Can you work these out from the model? Positions are in its coordinate system, mm. A direction names the side the tool comes from. Round coordinates to 2 decimals unless told otherwise and drop trailing zeros. Order: outer loops, then holes, each group sorted by start corner. A loop starts at its lowest first (then second) coordinate and runs counter-clockwise, first axis right, second up.
Q1. If I drill on line 1 (Y direction, x = 0, z = 0.6) (3 decimals); line 2 (X direction, y = 21.5, z = 5.5); line 3 (X direction, y = 8, z = 4.25), over which ranges is the centre line in solid material (lowest first)?
Q2. If we section it at D-D (y = 8): Please give me the cut outline in (x, z).
Q3. Will this pin go through, and if not, where does the flat tip stop? P1, Ø3.5, axis at x = -3.5, y = -24.5, coming from the +Z side.
Q4. For faces 1 (the face through (2, 23, 1)), 2 (the face through (0, -30.3, 6)), 3 (the face through (1, -32.5, 4)), which set-ups out of +Z, -Z, +X, -X, +Y, -Y let a thin tool reach every point of the face, with its end or its side?
Q5. If we section it at A-A (y = -24.5): Please give me the cut outline in (x, z).
Q6. If we section it at C-C (z = 6): Please give me the cut outline in (x, y), plus the area to 3 significant figures.
Q7. We'd pull the mould along X, two halves only. Please class faces 4 (the face through (12, 0, 6)), 5 (the face through (-1, 8, 0)), 6 (the face through (55, 0, 4)): pulls with the +X half, pulls with the -X half, needs draft (parallel to the pull), parting line crosses it, or undercut.
Q8. If we section it at B-B (x = 0): Please give me the cut outline in (y, z) (3 decimals).
Autodesk Inventor part; units mm, degrees
ref_plane "YZ Plane" through (0, 0, 0) normal (1, 0, 0) x (0, 1, 0)
ref_plane "XZ Plane" through (0, 0, 0) normal (0, 1, 0) x (-1, 0, 0)
ref_plane "XY Plane" through (0, 0, 0) normal (0, 0, 1) x (1, 0, 0)
sketch "Schizzo1" plane through (0, 0, 0) normal (0, 0, 1) x (1, 0, 0)
  line L0 (-55, 32.5) -> (55, 32.5)
  line L1 (55, 32.5) -> (55, -32.5)
  line L2 (55, -32.5) -> (-55, -32.5)
  line L3 (-55, -32.5) -> (-55, 32.5)
  line L4 (-55, 32.5) -> (55, -32.5) construction
  line L5 (55, 32.5) -> (-55, -32.5) construction
  line L6 (-8.5, -18.7) -> (8.5, -18.7)
  line L7 (8.5, -18.7) -> (8.5, -30.3)
  line L8 (8.5, -30.3) -> (-8.5, -30.3)
  line L9 (-8.5, -30.3) -> (-8.5, -18.7)
  line L10 (-8.5, -18.7) -> (8.5, -30.3) construction
  line L11 (8.5, -18.7) -> (-8.5, -30.3) construction
  line L12 (-12, 12) -> (12, 12)
  line L13 (12, 12) -> (12, -12)
  line L14 (12, -12) -> (-12, -12)
  line L15 (-12, -12) -> (-12, 12)
  line L16 (-12, 12) -> (12, -12) construction
  line L17 (12, 12) -> (-12, -12) construction
  line L18 (-8.95, 29.85) -> (8.95, 29.85)
  line L19 (8.95, 29.85) -> (8.95, 17)
  line L20 (8.95, 17) -> (-8.95, 17)
  line L21 (-8.95, 17) -> (-8.95, 29.85)
  line L22 (-8.95, 29.85) -> (8.95, 17) construction
  line L23 (8.95, 29.85) -> (-8.95, 17) construction
  line L24 (0, 25.425) -> (0, 21.425) construction
  line L25 (-2, 25.425) -> (-2, 21.425)
  line L26 (2, 21.425) -> (2, 25.425)
  arc A0 (2, 25.425) -> (-2, 25.425) centre (0, 25.425) ccw
  arc A1 (-2, 21.425) -> (2, 21.425) centre (0, 21.425) ccw
  circle A2 centre (0, -24.5) radius 4.1
  circle A3 centre (0, 0) radius 3.8
  line L27 (-4, 4) -> (4, 4)
  line L28 (4, 4) -> (4, -4)
  line L29 (4, -4) -> (-4, -4)
  line L30 (-4, -4) -> (-4, 4)
  line L31 (-4, 4) -> (4, -4) construction
  line L32 (4, 4) -> (-4, -4) construction
  point P0 (0, 23.425)
  dimension "d0" = 110
  dimension "d1" = 65
  dimension "d5" = 17
  dimension "d6" = 11.6
  dimension "d8" = 24
  dimension "d9" = 24
  dimension "d11" = 17.9
  dimension "d12" = 12.85
  dimension "d13" = 2
  dimension "d14" = 4
  dimension "d15" = 8.2
  dimension "d16" = 7.6
  dimension "d17" = 8
  dimension "d18" = 8
extrude "Estrusione1" add sketch "Schizzo1" along normal blind 9 contours L0 L1 L2 L3
sketch "Schizzo2" plane through (0, 0, 0) normal (0, 0, -1) x (-1, 0, 0)
  line L0 (-55, 32.5) -> (55, 32.5)
  line L1 (55, 32.5) -> (55, -32.5)
  line L2 (55, -32.5) -> (-55, -32.5)
  line L3 (-55, -32.5) -> (-55, 32.5)
  line L4 (-8.5, -18.7) -> (8.5, -18.7)
  line L5 (8.5, -18.7) -> (8.5, -30.3)
  line L6 (8.5, -30.3) -> (-8.5, -30.3)
  line L7 (-8.5, -30.3) -> (-8.5, -18.7)
  line L8 (-8.5, -18.7) -> (8.5, -30.3) construction
  line L9 (8.5, -18.7) -> (-8.5, -30.3) construction
  line L10 (-12, 12) -> (12, 12)
  line L11 (12, 12) -> (12, -12)
  line L12 (12, -12) -> (-12, -12)
  line L13 (-12, -12) -> (-12, 12)
  line L14 (-8.95, 29.85) -> (8.95, 29.85)
  line L15 (8.95, 29.85) -> (8.95, 17)
  line L16 (8.95, 17) -> (-8.95, 17)
  line L17 (-8.95, 17) -> (-8.95, 29.85)
  line L18 (-8.95, 29.85) -> (8.95, 17) construction
  line L19 (8.95, 29.85) -> (-8.95, 17) construction
  line L20 (0, 25.425) -> (0, 21.425) construction
  line L21 (-2, 25.425) -> (-2, 21.425)
  line L22 (2, 21.425) -> (2, 25.425)
  arc A0 (2, 25.425) -> (-2, 25.425) centre (0, 25.425) ccw
  arc A1 (-2, 21.425) -> (2, 21.425) centre (0, 21.425) ccw
  circle A2 centre (0, -24.5) radius 4.1
  line L23 (6.5, -6.5) -> (-6.5, -6.5)
  line L24 (-6.5, -6.5) -> (-6.5, 6.5)
  line L25 (-6.5, 6.5) -> (6.5, 6.5)
  line L26 (6.5, 6.5) -> (6.5, -6.5)
  point P0 (0, 0)
  point P1 (0, 0)
  point P2 (0, 23.425)
  dimension "d21" = 110
  dimension "d22" = 65
  dimension "d23" = 17
  dimension "d24" = 11.6
  dimension "d25" = 24
  dimension "d26" = 24
  dimension "d27" = 17.9
  dimension "d28" = 12.85
  dimension "d29" = 2
  dimension "d30" = 4
  dimension "d31" = 8.2
  dimension "d37" = 13
  dimension "d38" = 13
extrude "Estrusione4" add sketch "Schizzo2" against normal blind 2.5 contours L4 L5 L6 L7 | L10 L11 L12 L13 | L14 L15 L16 L17
Solution:
1. line 1: y = -32.5 to -28.6, -20.4 to -6.5, 6.5 to 19.425, 27.425 to 32.5
1. line 2: x = -55 to -8.95, 8.95 to 55
1. line 3: x = -55 to -12, 12 to 55
2. outline: (-55, 0) - (55, 0) - (55, 9) - (12, 9) - (12, 2.5) - (-12, 2.5) - (-12, 9) - (-55, 9) - close
3. P1: stops at z = 2.5
4. face 1: +Z, -Z
4. face 2: +Z
4. face 3: +Z, -Z, +X, -X, -Y
5. outline: (-55, 0) - (-4.1, 0) - (-4.1, 2.5) - (-8.5, 2.5) - (-8.5, 9) - (-55, 9) - close; (4.1, 0) - (55, 0) - (55, 9) - (8.5, 9) - (8.5, 2.5) - (4.1, 2.5) - close
6. outline: (-55, -32.5) - (55, -32.5) - (55, 32.5) - (-55, 32.5) - close; hole (-12, -12) - (12, -12) - (12, 12) - (-12, 12) - close; hole (-8.95, 17) - (8.95, 17) - (8.95, 29.85) - (-8.95, 29.85) - close; hole (-8.5, -30.3) - (8.5, -30.3) - (8.5, -18.7) - (-8.5, -18.7) - close
6. area: 6,150 mm2
7. face 4: undercut
7. face 5: needs draft
7. face 6: pulls with the +X half
8. outline: (-32.5, 0) - (-28.6, 0) - (-28.6, 2.5) - (-30.3, 2.5) - (-30.3, 9) - (-32.5, 9) - close; (-20.4, 0) - (-6.5, 0) - (-6.5, 2.5) - (-12, 2.5) - (-12, 9) - (-18.7, 9) - (-18.7, 2.5) - (-20.4, 2.5) - close; (6.5, 0) - (19.425, 0) - (19.425, 2.5) - (17, 2.5) - (17, 9) - (12, 9) - (12, 2.5) - (6.5, 2.5) - close; (27.425, 0) - (32.5, 0) - (32.5, 9) - (29.85, 9) - (29.85, 2.5) - (27.425, 2.5) - close
